The model under review builds one solid part; all positions refer to its coordinate system, in mm. Face numbers are marked on the shaded views. Give positions to 0.01 mm unless a question says otherwise; leave off trailing zeros. Order: outer loops, then holes, each group sorted by start corner. A loop starts at its lowest first (then second) coordinate and runs counter-clockwise, first axis right, second up.
```python
from build123d import *

# Parameters (mm, degrees)
F0_R     = 100
F0_R_2   = 2.5
F0_R_3   = 6.86
F0_W     = 100
F0_H     = 100
F1_DEPTH = 5


with BuildPart() as f1:
    # F0 (on Top) → F1 (new body)
    with BuildSketch(Plane.XY):
        Circle(F0_R)
        with Locations((-52.5, -52.5)):
            Circle(F0_R_2, mode=Mode.SUBTRACT)
        with Locations((-83.149158, -34.441509)):
            Circle(F0_R_3, mode=Mode.SUBTRACT)
        with Locations((0, -80)):
            Circle(F0_R_2, mode=Mode.SUBTRACT)
        with Locations((52.5, -52.5)):
            Circle(F0_R_2, mode=Mode.SUBTRACT)
        with Locations((83.149158, -34.441509)):
            Circle(F0_R_3, mode=Mode.SUBTRACT)
        with Locations((-80, 0)):
            Circle(F0_R_2, mode=Mode.SUBTRACT)
        with Locations((-52.5, 52.5)):
            Circle(F0_R_2, mode=Mode.SUBTRACT)
        with Locations((-54.788529, 71.401801)):
            Circle(F0_R_3, mode=Mode.SUBTRACT)
        Rectangle(F0_W, F0_H, mode=Mode.SUBTRACT)
        with Locations((80, 0)):
            Circle(F0_R_2, mode=Mode.SUBTRACT)
        with Locations((0, 80)):
            Circle(F0_R_2, mode=Mode.SUBTRACT)
        with Locations((52.5, 52.5)):
            Circle(F0_R_2, mode=Mode.SUBTRACT)
        with Locations((54.788529, 71.401801)):
            Circle(F0_R_3, mode=Mode.SUBTRACT)
    extrude(amount=F1_DEPTH)


solid = f1.part
```
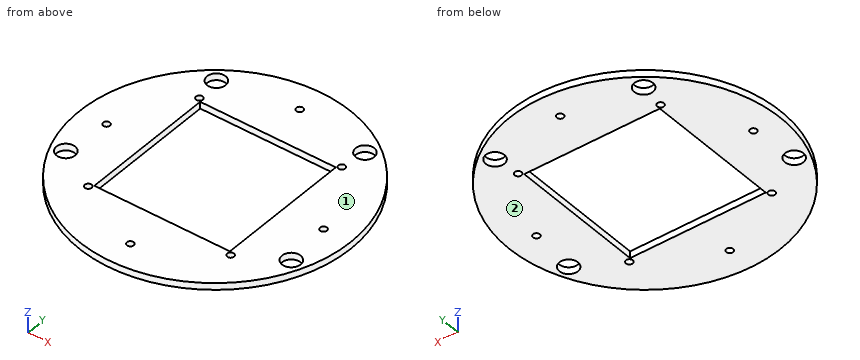
Item 1: For line 1 (Y direction, x = 0, z = 3.3); line 2 (Y direction, x = 52.5, z = 2.75); line 3 (Y direction, x = 80, z = 3.4), list the stretches that pass through material, from the lowest coordinate up.
Values found:
line 1: y = -100 to -82.5, -77.5 to -50, 50 to 77.5, 82.5 to 100
line 2: y = -85.11 to -55, -50 to 50, 55 to 64.93, 77.87 to 85.11
line 3: y = -60 to -40.54, -28.35 to -2.5, 2.5 to 60
Item 2: Take a section at C-C (y = -80). Give the boundary of the cut face in (x, z).
Values found:
outline: (-60, 0) - (-2.5, 0) - (-2.5, 5) - (-60, 5) - close; (2.5, 0) - (60, 0) - (60, 5) - (2.5, 5) - close
Item 3: Clearance check with flat-ended pins moving along their axes: pin 1 Ø2 at (x, y) = (-30, -62) entering from -Z; pin 2 Ø1.5 at (y, z) = (-59, 2) entering from -X; pin 3 Ø2.5 at (y, z) = (-17, 1.5) entering from +X. State where each tip first meets the part, or that it passes through.
Values found:
pin 1: stops at z = 0
pin 2: stops at x = -81.28
pin 3: stops at x = 98.75
Item 4: Take a section at A-A (y = 0). Give the boundary of the cut face in (x, z), and give its area (3 significant figures).
Values found:
outline: (-100, 0) - (-82.5, 0) - (-82.5, 5) - (-100, 5) - close; (-77.5, 0) - (-50, 0) - (-50, 5) - (-77.5, 5) - close; (50, 0) - (77.5, 0) - (77.5, 5) - (50, 5) - close; (82.5, 0) - (100, 0) - (100, 5) - (82.5, 5) - close
area: 450 mm2
Item 5: Draft analysis for pull direction Z (two halves, no side actions). For the marked faces 1 and 2, state which applies: released by +Z, released by -Z, zero draft, split by the parting line, or undercut.
Values found:
face 1: released by +Z
face 2: released by -Z
Item 6: Take a section at D-D (z = 2.95). Give the number of separate pieces and of enclosed holes in the cut face, and give its area (3 significant figures).
Values found:
separate pieces: 1
enclosed holes: 13
area: 20,700 mm2
